Here's how the part is built. I have some questions about the finished solid (model axes, mm). Face numbers are marked on the shaded views. A direction names the side the tool comes from. Coordinates: 2 decimals unless noted, no trailing zeros. Write each loop counter-clockwise with the first axis right and the second up, starting at its lowest first coordinate (ties: lowest second). Pieces come first, ordered by that corner, then holes.
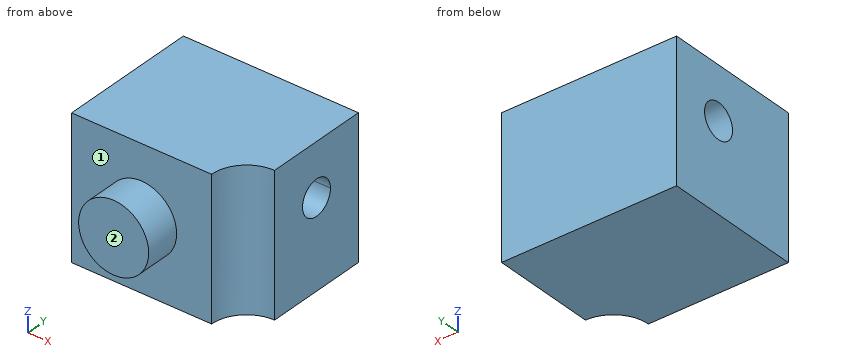
from build123d import *

# Parameters (mm, degrees)
F0_W     = 5
F0_H     = 4
F1_DEPTH = 4
F4_R     = 1
F5_DEPTH = 25
F6_R     = 1
F7_DEPTH = 1
F9_DEPTH = 25


with BuildPart() as f1:
    # F0 (on Top) → F1 (new body)
    with BuildSketch(Plane.XY):
        with Locations((2.5, 2)):
            Rectangle(F0_W, F0_H)
    extrude(amount=F1_DEPTH)

    # F4 (on face) → F5 (cut)
    with BuildSketch(Plane.XY.offset(4)):
        with Locations((5, 0)):
            Circle(F4_R)
    extrude(amount=-F5_DEPTH, mode=Mode.SUBTRACT)

    # F6 (on face) → F7 (join)
    with BuildSketch(Plane.XZ):
        with Locations((2, 2)):
            Circle(F6_R)
    extrude(amount=F7_DEPTH)

    # F8 (on face) → F9 (cut)
    with BuildSketch(Plane.YZ.offset(5)):
        with BuildLine():
            ThreePointArc((3, 2.5), (2.96194, 2.691342), (2.853553, 2.853553))
            Line((2.853553, 2.853553), (2.146447, 2.146447))
            ThreePointArc((2.146447, 2.146447), (2.691342, 2.03806), (3, 2.5))
        make_face()
        with BuildLine():
            Line((2.146447, 2.146447), (2.853553, 2.853553))
            ThreePointArc((2.853553, 2.853553), (2.146447, 2.853553), (2.146447, 2.146447))
        make_face()
    extrude(amount=-F9_DEPTH, mode=Mode.SUBTRACT)


solid = f1.part
1. If I drill on line 1 (Y direction, x = 0.25, z = 3.75); line 2 (Y direction, x = 3.65, z = 2.3); line 3 (Y direction, x = 4.55, z = 0.4), over which ranges is the centre line in solid material (lowest first)?
2. On a 3-axis mill with a long thin cutter (end or side, diameter ignored), from which of +Z, -Z, +X, -X, +Y, -Y can I reach the whole of each face in a straight line? I mean the marked faces 1 and 2. Say none if no direction works.
3. I want a section at D-D (y = 0.5). List the corners of the cut face in (x, z) for me.
4. I want a section at A-A (y = 2.5). List the corners of the cut face in (x, z) for me, then the cut area to 3 significant figures.
5. I want a section at B-B (x = 3.25). List the corners of the cut face in (y, z) for me, then the cut area to 3 significant figures.
6. I want a section at C-C (x = 2). List the corners of the cut face in (y, z) for me.
7. For pin 1 Ø1 at (x, z) = (3.5, 2.5) entering from -Y, with a flat end and sliding along its axis, tell me the tip position at first contact or that it passes through.
Response values:
1. line 1: y = 0 to 4
1. line 2: y = 0 to 2.04, 2.96 to 4
1. line 3: y = 0.89 to 4
2. face 1: -Y
2. face 2: +Z, -Z, +X, -X, -Y
3. outline: (0, 0) - (4.13, 0) - (4.13, 4) - (0, 4) - close
4. outline: (0, 0) - (5, 0) - (5, 2) - (0, 2) - close; (0, 3) - (5, 3) - (5, 4) - (0, 4) - close
4. area: 15.0 mm2
5. outline: (0, 0) - (4, 0) - (4, 4) - (0, 4) - close; hole (2.85, 2.85) arc R0.5 ccw (long way) to (3, 2.5) arc R0.5 ccw to start
5. area: 15.2 mm2
6. outline: (-1, 1) - (0, 1) - (0, 0) - (4, 0) - (4, 4) - (0, 4) - (0, 3) - (-1, 3) - close; hole (2.85, 2.85) arc R0.5 ccw (long way) to (3, 2.5) arc R0.5 ccw to start
7. pin 1: stops at y = 0
